Autodesk Inventor part; units mm, degrees
ref_plane "YZ Plane" through (0, 0, 0) normal (1, 0, 0) x (0, 1, 0)
ref_plane "XZ Plane" through (0, 0, 0) normal (0, 1, 0) x (-1, 0, 0)
ref_plane "XY Plane" through (0, 0, 0) normal (0, 0, 1) x (1, 0, 0)
sketch "Sketch1" plane through (0, 0, 0) normal (0, 1, 0) x (-1, 0, 0)
  circle A0 centre (0, 0) radius 4
  circle A1 centre (0, 0) radius 3
extrude "Extrusion1" add sketch "Sketch1" along normal blind 3
fillet "Fillet1" radius 0.5 1 edges at (3, 3, 0)
fillet "Fillet2" radius 0.5 1 edges at (4, 3, 0)
properties part number "Chimera Hetsink Brass Insert" material "Brass"
Read the model definition and answer for the solid it produces. Units are mm, in the model's axes. Round coordinates to 2 decimals unless told otherwise and drop trailing zeros. Write each loop counter-clockwise with the first axis right and the second up, starting at its lowest first coordinate (ties: lowest second). Pieces come first, ordered by that corner, then holes.
Q1. The mould has two halves that part along Z. Classify faces 1 (the face through (3, 1, 0)), 2 (the face through (-1, 0, 3)), 3 (the face through (0.867, 1.233, 3.905)): released by +Z, released by -Z, zero draft, split by the parting line, or undercut.
Values:
face 1: undercut
face 2: zero draft
face 3: split by the parting line
Q2. A flat-ended cylindrical pin translates along its axis: P1, Ø4, axis at x = 1, z = 1, coming from the +Y side. Find the tip coordinate at first contact, or state that the pin passes through.
Values:
P1: stops at y = 2.99
Q3. Find section D-D on y = 2.7. Determine the outline of the cut face in (x, z), and give its area (3 significant figures).
Values:
outline: circle Ø7.92 at (0, 0); hole circle Ø6.08 at (0, 0)
area: 20.2 mm2
Q4. Straight lines are drawn through the part: line 1 (Z direction, x = 0, y = 0.65); line 2 (X direction, y = 0.75, z = 2); line 3 (X direction, y = 1.5, z = -0.75). For each, find the intervals that lie inside material, in ascending order.
Values:
line 1: z = -4 to -3, 3 to 4
line 2: x = -3.46 to -2.24, 2.24 to 3.46
line 3: x = -3.93 to -2.9, 2.9 to 3.93
Q5. Find section C-C on y = 0.5. Determine the outline of the cut face in (x, z), and give its area (3 significant figures).
Values:
outline: circle Ø8 at (0, 0); hole circle Ø6 at (0, 0)
area: 22.0 mm2
